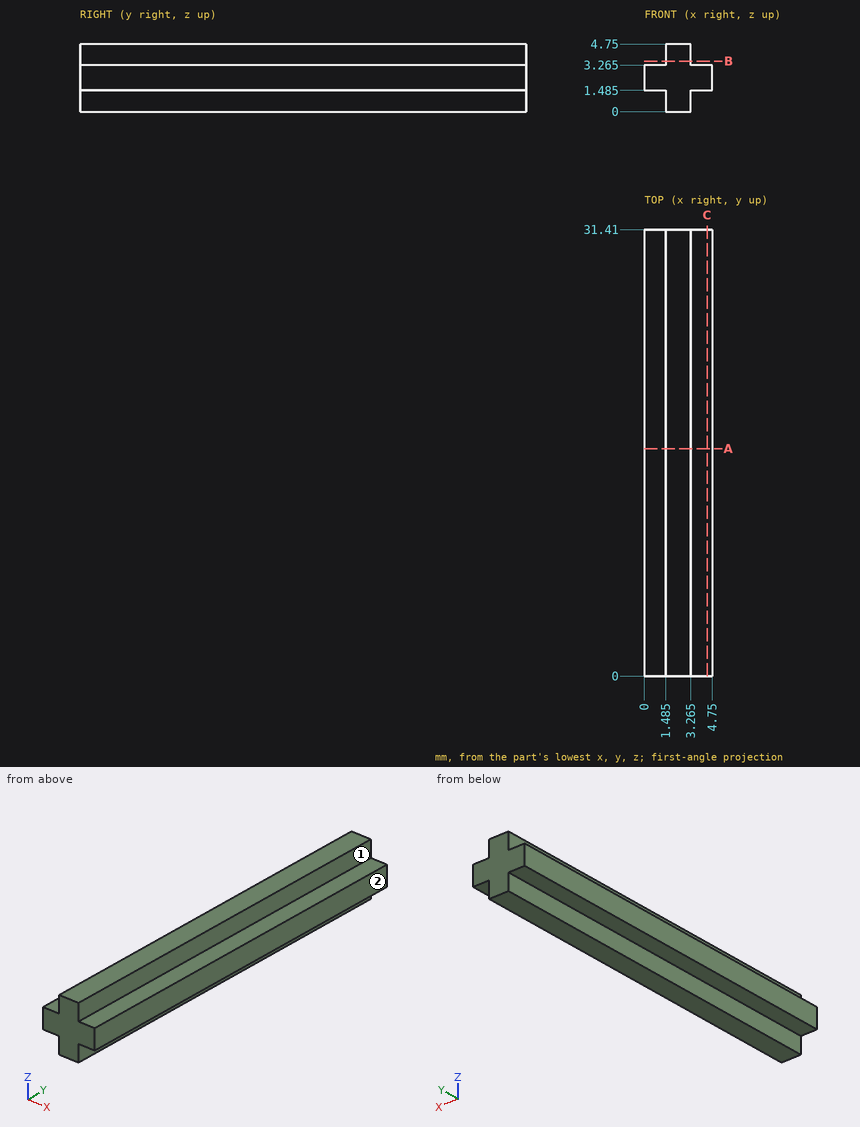
Study the drawing (mm; zero at the part's minimum x, y, z) and answer. A direction names the side the tool comes from. Coordinates: 2 decimals unless noted, no trailing zeros. Write each loop counter-clockwise with the first axis right and the second up, starting at its lowest first coordinate (ties: lowest second). Pieces come first, ordered by that corner, then holes.
Q1. Which of the six approach directions +Z, -Z, +X, -X, +Y, -Y give full straight-line access (tool end or side, diameter ignored) to the marked faces 1 and 2?
Returned:
face 1: +Z, +X, +Y, -Y
face 2: +Z, -Z, +X, +Y, -Y
Q2. Section C-C, the plane x = 4.4 is taken. Write down the section's boundary in (y, z) (3 decimals), then the cut area to 3 significant figures.
Returned:
outline: (0, 1.485) - (31.41, 1.485) - (31.41, 3.265) - (0, 3.265) - close
area: 55.9 mm2
Q3. Find the intervals of material crossed by line 1 along Z through (x, y) = (0.8, 7.5) (3 decimals), in increasing order.
Returned:
line 1: z = 1.485 to 3.265
Q4. Given P1, Ø1.2, axis at x = 4, y = 8.5, coming from the -Z side (3 decimals); P2, Ø1.2, axis at y = 21, z = 0.5, coming from the +X side (3 decimals); P3, Ø0.7, axis at x = 4, y = 22, coming from the +Z side (3 decimals), each flat-ended and moving along its own axis, determine where each tip first touches the part or whether it passes through.
Returned:
P1: stops at z = 1.485
P2: stops at x = 3.265
P3: stops at z = 3.265
Q5. Section A-A, the plane y = 16 is taken. Write down the section's boundary in (x, z) (3 decimals), then the cut area to 3 significant figures.
Returned:
outline: (0, 1.485) - (1.485, 1.485) - (1.485, 0) - (3.265, 0) - (3.265, 1.485) - (4.75, 1.485) - (4.75, 3.265) - (3.265, 3.265) - (3.265, 4.75) - (1.485, 4.75) - (1.485, 3.265) - (0, 3.265) - close
area: 13.7 mm2
Q6. Section B-B, the plane z = 3.55 is taken. Write down the section's boundary in (x, y) (3 decimals).
Returned:
outline: (1.485, 0) - (3.265, 0) - (3.265, 31.41) - (1.485, 31.41) - close
